```python
from build123d import *

# Parameters (mm, degrees)
F0_W         = 17.52
F0_H         = 17.52
F0_H_2       = 17.57
F0_R         = 1.5
F1_DEPTH     = 1
F2_W         = 17.52
F2_H         = 17.57
F2_H_2       = 17.52
F3_DEPTH     = 1
F4_R         = 3.5
F5_DEPTH     = 0.5
F6_R         = 4.25
F6_R_2       = 3.5
F7_DEPTH     = 0.25
F8_T1_DEPTH  = 32.52
F8_T3_DEPTH  = 32.52
F8_T5_DEPTH  = 32.57
F8_T7_DEPTH  = 32.52
F8_T12_DEPTH = 32.52
F8_S13_R     = 4.25
F8_T14_DEPTH = 18
F8_T18_DEPTH = 32.52
F8_S19_R     = 4.25
F8_T20_DEPTH = 18
F8_T24_DEPTH = 32.52
F8_S25_R     = 4.25
F8_T26_DEPTH = 18
F8_T30_DEPTH = 32.57
F8_S31_R     = 4.25
F8_T32_DEPTH = 18
F8_T36_DEPTH = 32.57
F8_S37_R     = 4.25
F8_T38_DEPTH = 18
F8_T42_DEPTH = 32.52
F8_S43_R     = 4.25
F8_T44_DEPTH = 18
F8_T48_DEPTH = 32.52
F8_S49_R     = 4.25
F8_T50_DEPTH = 18
F8_T54_DEPTH = 32.52
F8_S55_R     = 4.25
F8_T56_DEPTH = 18
F9_R         = 1.05
F10_DEPTH    = 0.5


# Not quite as in the source:
# - a fillet or chamfer that OpenCascade refuses, or shapes differently, is made with other operations: its cross-section is extruded or revolved along the edge and cut away or added


with BuildPart() as f1:
    # F0 (on Top) → F1 (new body)
    with BuildSketch(Plane.XY):
        with BuildLine():
            ThreePointArc((-25, -24), (-24.7071067812, -24.7071067812), (-24, -25))
            Line((-24, -25), (-15.1855654437, -25))
            ThreePointArc((-15.1855654437, -25), (-14.2350281943, -24.0494627506), (-13.2844909448, -25))
            Line((-13.2844909448, -25), (13.2844909448, -25))
            ThreePointArc((13.2844909448, -25), (14.2350281943, -24.0494627506), (15.1855654437, -25))
            Line((15.1855654437, -25), (24, -25))
            ThreePointArc((24, -25), (24.7071067812, -24.7071067812), (25, -24))
            Line((25, -24), (25, 22.7180756629))
            Line((25, 22.7180756629), (22.7180756629, 25))
            Line((22.7180756629, 25), (15.1855654437, 25))
            ThreePointArc((15.1855654437, 25), (14.2350281943, 24.0494627506), (13.2844909448, 25))
            Line((13.2844909448, 25), (4.4700563885, 25))
            Line((4.4700563885, 25), (3.8659917191, 24.0494627506))
            Line((3.8659917191, 24.0494627506), (0, 24.0494627506))
            Line((0, 24.0494627506), (-3.8659917191, 24.0494627506))
            Line((-3.8659917191, 24.0494627506), (-4.4700563885, 25))
            Line((-4.4700563885, 25), (-13.2844909448, 25))
            ThreePointArc((-13.2844909448, 25), (-14.2350281943, 24.0494627506), (-15.1855654437, 25))
            Line((-15.1855654437, 25), (-24, 25))
            ThreePointArc((-24, 25), (-24.7071067812, 24.7071067812), (-25, 24))
            Line((-25, 24), (-25, -24))
        make_face()
        with Locations((-12.26, -12.26)):
            Rectangle(F0_W, F0_H, mode=Mode.SUBTRACT)
        with Locations((12.26, -12.26)):
            Rectangle(F0_W, F0_H, mode=Mode.SUBTRACT)
        with Locations((-12.26, 12.285)):
            Rectangle(F0_W, F0_H_2, mode=Mode.SUBTRACT)
        Circle(F0_R, mode=Mode.SUBTRACT)
        with Locations((12.26, 12.285)):
            Rectangle(F0_W, F0_H_2, mode=Mode.SUBTRACT)
    extrude(amount=F1_DEPTH)

    # F2 (on face) → F3 (join, symmetric)
    with BuildSketch(Plane.XY.offset(1)):
        with Locations((-12.26, 12.285)):
            Rectangle(F2_W, F2_H)
        with Locations((12.26, 12.285)):
            Rectangle(F2_W, F2_H)
        with Locations((12.26, -12.26)):
            Rectangle(F2_W, F2_H_2)
        with Locations((-12.26, -12.26)):
            Rectangle(F2_W, F2_H_2)
    extrude(amount=F3_DEPTH, both=True)

    # F4 (on face) → F5 (cut)
    with BuildSketch(Plane.XY.offset(1)):
        Circle(F4_R)
    extrude(amount=-F5_DEPTH, mode=Mode.SUBTRACT)

    # F6 (on face) → F7 (join)
    with BuildSketch(Plane.XY.offset(1)):
        Circle(F6_R)
        Circle(F6_R_2, mode=Mode.SUBTRACT)
    extrude(amount=F7_DEPTH)

    # F8: fillet of radius 5 on 16 edges, made by hand

    # F8_s2 → F8_t1 (cut)
    with BuildSketch(Plane.YZ.offset(-28.52)):
        with BuildLine():
            ThreePointArc((-21.02, 1), (-19.6011388301, 1.7434164903), (-18.02, 2))
            Line((-18.02, 2), (-21.02, 2))
            Line((-21.02, 2), (-21.02, 1))
        make_face()
        with BuildLine():
            ThreePointArc((21.07, 1), (19.6511388301, 1.7434164903), (18.07, 2))
            Line((18.07, 2), (21.07, 2))
            Line((21.07, 2), (21.07, 1))
        make_face()
    extrude(amount=F8_T1_DEPTH, mode=Mode.SUBTRACT)

    # F8_s4 → F8_t3 (cut)
    with BuildSketch(Plane.XZ.offset(-4)):
        with BuildLine():
            ThreePointArc((-21.02, 1), (-19.6011388301, 1.7434164903), (-18.02, 2))
            Line((-18.02, 2), (-21.02, 2))
            Line((-21.02, 2), (-21.02, 1))
        make_face()
        with BuildLine():
            ThreePointArc((21.02, 1), (19.6011388301, 1.7434164903), (18.02, 2))
            Line((18.02, 2), (21.02, 2))
            Line((21.02, 2), (21.02, 1))
        make_face()
    extrude(amount=F8_T3_DEPTH, mode=Mode.SUBTRACT)

    # F8_s6 → F8_t5 (cut)
    with BuildSketch(Plane.XZ.offset(-28.57)):
        with BuildLine():
            ThreePointArc((-21.02, 1), (-19.6011388301, 1.7434164903), (-18.02, 2))
            Line((-18.02, 2), (-21.02, 2))
            Line((-21.02, 2), (-21.02, 1))
        make_face()
        with BuildLine():
            ThreePointArc((21.02, 1), (19.6011388301, 1.7434164903), (18.02, 2))
            Line((18.02, 2), (21.02, 2))
            Line((21.02, 2), (21.02, 1))
        make_face()
    extrude(amount=F8_T5_DEPTH, mode=Mode.SUBTRACT)

    # F8_s8 → F8_t7 (cut)
    with BuildSketch(Plane.YZ.offset(-4)):
        with BuildLine():
            ThreePointArc((21.07, 1), (19.6511388301, 1.7434164903), (18.07, 2))
            Line((18.07, 2), (21.07, 2))
            Line((21.07, 2), (21.07, 1))
        make_face()
        with BuildLine():
            ThreePointArc((-21.02, 1), (-19.6011388301, 1.7434164903), (-18.02, 2))
            Line((-18.02, 2), (-21.02, 2))
            Line((-21.02, 2), (-21.02, 1))
        make_face()
    extrude(amount=F8_T7_DEPTH, mode=Mode.SUBTRACT)


with BuildPart() as f8_tool10:
    # F8_s11 → F8_t12 (new body)
    with BuildSketch(Plane.XZ.offset(28.52)):
        with BuildLine():
            ThreePointArc((-3.5, 1), (-4.9188611699, 1.7434164903), (-6.5, 2))
            Line((-6.5, 2), (-3.5, 2))
            Line((-3.5, 2), (-3.5, 1))
        make_face()
    extrude(amount=-F8_T12_DEPTH)

    # F8_s13 → F8_t14 (cut, symmetric)
    with BuildSketch(Plane.XY.offset(1.5)):
        Circle(F8_S13_R)
    extrude(amount=F8_T14_DEPTH, both=True, mode=Mode.SUBTRACT)


with BuildPart() as f1_1:
    add(f1.part)

    # F8_t9: cut F8_tool10
    add(f8_tool10.part, mode=Mode.SUBTRACT)


with BuildPart() as f8_tool16:
    # F8_s17 → F8_t18 (new body)
    with BuildSketch(Plane.YZ.offset(4)):
        with BuildLine():
            ThreePointArc((-3.5, 1), (-4.9188611699, 1.7434164903), (-6.5, 2))
            Line((-6.5, 2), (-3.5, 2))
            Line((-3.5, 2), (-3.5, 1))
        make_face()
    extrude(amount=-F8_T18_DEPTH)

    # F8_s19 → F8_t20 (cut, symmetric)
    with BuildSketch(Plane.XY.offset(1.5)):
        Circle(F8_S19_R)
    extrude(amount=F8_T20_DEPTH, both=True, mode=Mode.SUBTRACT)


with BuildPart() as f1_2:
    add(f1_1.part)

    # F8_t15: cut F8_tool16
    add(f8_tool16.part, mode=Mode.SUBTRACT)


with BuildPart() as f8_tool22:
    # F8_s23 → F8_t24 (new body)
    with BuildSketch(Plane.YZ.offset(-28.52)):
        with BuildLine():
            ThreePointArc((3.5, 1), (4.9188611699, 1.7434164903), (6.5, 2))
            Line((6.5, 2), (3.5, 2))
            Line((3.5, 2), (3.5, 1))
        make_face()
    extrude(amount=F8_T24_DEPTH)

    # F8_s25 → F8_t26 (cut, symmetric)
    with BuildSketch(Plane.XY.offset(1.5)):
        Circle(F8_S25_R)
    extrude(amount=F8_T26_DEPTH, both=True, mode=Mode.SUBTRACT)


with BuildPart() as f1_3:
    add(f1_2.part)

    # F8_t21: cut F8_tool22
    add(f8_tool22.part, mode=Mode.SUBTRACT)


with BuildPart() as f8_tool28:
    # F8_s29 → F8_t30 (new body)
    with BuildSketch(Plane.XZ.offset(4)):
        with BuildLine():
            ThreePointArc((-3.5, 1), (-4.9188611699, 1.7434164903), (-6.5, 2))
            Line((-6.5, 2), (-3.5, 2))
            Line((-3.5, 2), (-3.5, 1))
        make_face()
    extrude(amount=-F8_T30_DEPTH)

    # F8_s31 → F8_t32 (cut, symmetric)
    with BuildSketch(Plane.XY.offset(1.5)):
        Circle(F8_S31_R)
    extrude(amount=F8_T32_DEPTH, both=True, mode=Mode.SUBTRACT)


with BuildPart() as f1_4:
    add(f1_3.part)

    # F8_t27: cut F8_tool28
    add(f8_tool28.part, mode=Mode.SUBTRACT)


with BuildPart() as f8_tool34:
    # F8_s35 → F8_t36 (new body)
    with BuildSketch(Plane.XZ.offset(-28.57)):
        with BuildLine():
            ThreePointArc((3.5, 1), (4.9188611699, 1.7434164903), (6.5, 2))
            Line((6.5, 2), (3.5, 2))
            Line((3.5, 2), (3.5, 1))
        make_face()
    extrude(amount=F8_T36_DEPTH)

    # F8_s37 → F8_t38 (cut, symmetric)
    with BuildSketch(Plane.XY.offset(1.5)):
        Circle(F8_S37_R)
    extrude(amount=F8_T38_DEPTH, both=True, mode=Mode.SUBTRACT)


with BuildPart() as f1_5:
    add(f1_4.part)

    # F8_t33: cut F8_tool34
    add(f8_tool34.part, mode=Mode.SUBTRACT)


with BuildPart() as f8_tool40:
    # F8_s41 → F8_t42 (new body)
    with BuildSketch(Plane.YZ.offset(-4)):
        with BuildLine():
            ThreePointArc((3.5, 1), (4.9188611699, 1.7434164903), (6.5, 2))
            Line((6.5, 2), (3.5, 2))
            Line((3.5, 2), (3.5, 1))
        make_face()
    extrude(amount=F8_T42_DEPTH)

    # F8_s43 → F8_t44 (cut, symmetric)
    with BuildSketch(Plane.XY.offset(1.5)):
        Circle(F8_S43_R)
    extrude(amount=F8_T44_DEPTH, both=True, mode=Mode.SUBTRACT)


with BuildPart() as f1_6:
    add(f1_5.part)

    # F8_t39: cut F8_tool40
    add(f8_tool40.part, mode=Mode.SUBTRACT)


with BuildPart() as f8_tool46:
    # F8_s47 → F8_t48 (new body)
    with BuildSketch(Plane.YZ.offset(28.52)):
        with BuildLine():
            ThreePointArc((-3.5, 1), (-4.9188611699, 1.7434164903), (-6.5, 2))
            Line((-6.5, 2), (-3.5, 2))
            Line((-3.5, 2), (-3.5, 1))
        make_face()
    extrude(amount=-F8_T48_DEPTH)

    # F8_s49 → F8_t50 (cut, symmetric)
    with BuildSketch(Plane.XY.offset(1.5)):
        Circle(F8_S49_R)
    extrude(amount=F8_T50_DEPTH, both=True, mode=Mode.SUBTRACT)


with BuildPart() as f1_7:
    add(f1_6.part)

    # F8_t45: cut F8_tool46
    add(f8_tool46.part, mode=Mode.SUBTRACT)


with BuildPart() as f8_tool52:
    # F8_s53 → F8_t54 (new body)
    with BuildSketch(Plane.XZ.offset(-4)):
        with BuildLine():
            ThreePointArc((3.5, 1), (4.9188611699, 1.7434164903), (6.5, 2))
            Line((6.5, 2), (3.5, 2))
            Line((3.5, 2), (3.5, 1))
        make_face()
    extrude(amount=F8_T54_DEPTH)

    # F8_s55 → F8_t56 (cut, symmetric)
    with BuildSketch(Plane.XY.offset(1.5)):
        Circle(F8_S55_R)
    extrude(amount=F8_T56_DEPTH, both=True, mode=Mode.SUBTRACT)


with BuildPart() as f1_8:
    add(f1_7.part)

    # F8_t51: cut F8_tool52
    add(f8_tool52.part, mode=Mode.SUBTRACT)

    # F9 (on face) → F10 (join)
    with BuildSketch(Plane(origin=(0, 0, 0), x_dir=(1, 0, 0), z_dir=(0, 0, -1))):
        with Locations((0, 22.5)):
            Circle(F9_R)
        with Locations((0, -22.5)):
            Circle(F9_R)
    extrude(amount=F10_DEPTH)


solid = f1_8.part
```
Source: CAD feature listing. Evaluate the final solid. Frame: model axes, mm. A direction names the side the tool comes from. Coordinates: 2 decimals unless noted, no trailing zeros. Loops run counter-clockwise (first coordinate to the right, second up) from the corner with the lowest first, then second, coordinate; pieces in that order, holes last. Notation, with made-up numbers: M 43.25,64.25 L 69.25,64.25 A15 cw 69.25,74.25 Z; hole C -37.75,-16.75 d3. An arc over 180 degrees is marked long. Put each result on its own line as item: value. Start each with the question number.
1) Ray query, L1, parallel to Y at x = 0, z = 0.85; L2, parallel to Y at x = 0, z = 0.35; L3, parallel to X at y = 0, z = 0.2. Return the intervals inside material, ascending. Write a range as from..to.
2) Pull-direction query (Y, two-part tool) for faces 4 (the face through (0, -23, -0.5)), 5 (the face through (-6, 0, 1)), 6 (the face through (12.137, 19.672, 1.736)); classes: pulls with the +Y half, pulls with the -Y half, needs draft (parallel to the pull), parting line crosses it, or undercut.
3) Reachability of faces 1 (the face through (4.898, 12.408, 1.736)), 2 (the face through (0, -2, 0.5)), 3 (the face through (12.383, -4.898, 1.736)) from +Z, -Z, +X, -X, +Y, -Y: full face, straight path, thin tool, end or side. Return the list, or none.
4) Cut plane A-A on x = 0. Return the cut outline in (y, z), then the cut area to 3 significant figures.
5) Contact query for flat-ended pins moving along their axis: pin 1 Ø0.8 at (x, z) = (-0.5, 0.5) entering from +Y; pin 2 Ø25 at (x, y) = (7, -2.5) entering from -Z; pin 3 Ø1.5 at (x, y) = (-1, 5.5) entering from +Z. Output: stop coordinate, or through.
6) Cut plane D-D on x = 14. Return the cut outline in (y, z).
7) Cut plane C-C on y = -22.5. Return the cut outline in (x, z).
8) Cut plane B-B on y = 0. Return the cut outline in (x, z).
The answers:
1. L1: y = -25..-3.5, 3.5..24.05
1. L2: y = -25..-1.5, 1.5..24.05
1. L3: x = -25..-1.5, 1.5..25
2. face 4: needs draft
2. face 5: undercut
2. face 6: pulls with the +Y half
3. face 1: +Z, +Y
3. face 2: +Z
3. face 3: +Z, +X
4. outline: M -25,0 L -23.55,0 L -23.55,-0.5 L -21.45,-0.5 L -21.45,0 L -1.5,0 L -1.5,0.5 L -3.5,0.5 L -3.5,1.25 L -4.25,1.25 L -4.25,1 L -25,1 Z; M 1.5,0 L 21.45,0 L 21.45,-0.5 L 23.55,-0.5 L 23.55,0 L 24.05,0 L 24.05,1 L 4.25,1 L 4.25,1.25 L 3.5,1.25 L 3.5,0.5 L 1.5,0.5 Z
4. area: 46.5 mm²
5. pin 1: stops at y = 24.05
5. pin 2: stops at z = 0
5. pin 3: stops at z = 1
6. outline: M -24.08,0 L 24.08,0 L 24.08,1 L 21.07,1 A5 ccw 18.07,2 L 6.5,2 A5 ccw 3.5,1 L -3.5,1 A5 ccw -6.5,2 L -18.02,2 A5 ccw -21.02,1 L -24.08,1 Z
7. outline: M -25,0 L -1.05,0 L -1.05,-0.5 L 1.05,-0.5 L 1.05,0 L 25,0 L 25,1 L -25,1 Z
8. outline: M -25,0 L -1.5,0 L -1.5,0.5 L -3.5,0.5 L -3.5,1.25 L -4.25,1.25 L -4.25,1 L -25,1 Z; M 1.5,0 L 25,0 L 25,1 L 4.25,1 L 4.25,1.25 L 3.5,1.25 L 3.5,0.5 L 1.5,0.5 Z
